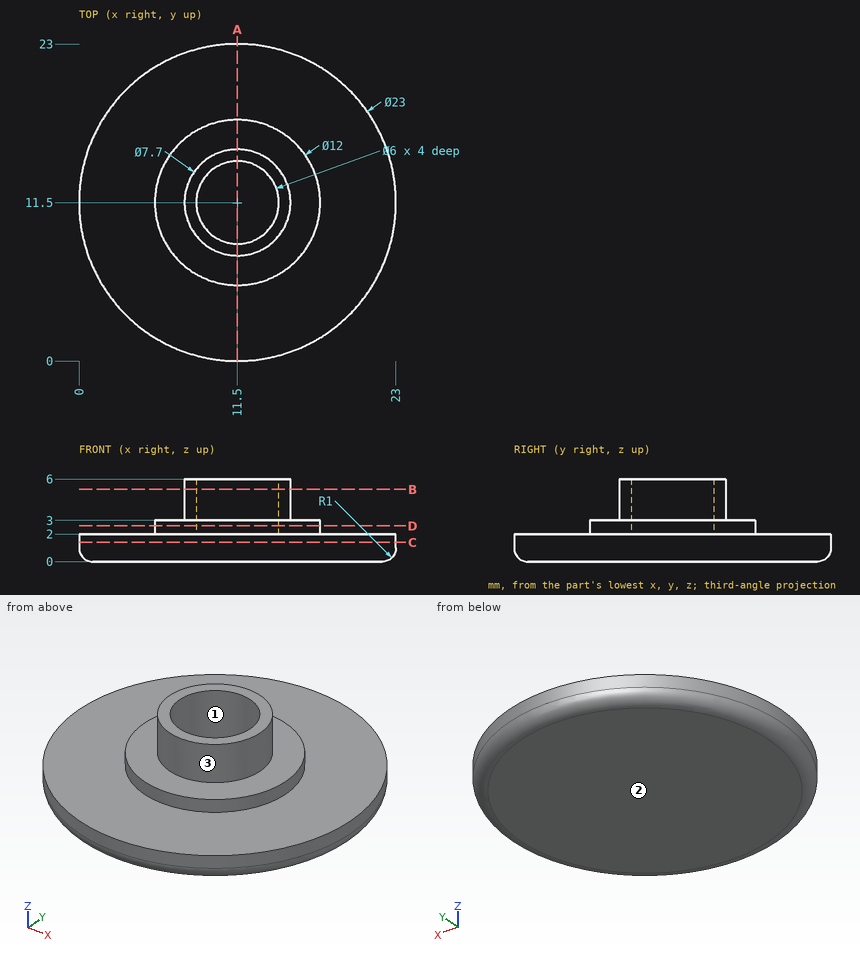
Design review of the part shown in the three views and the two pictorial views. Dimensions are in mm from the part's minimum x, y and z. Give positions to 0.01 mm unless a question says otherwise; leave off trailing zeros. Loops run counter-clockwise (first coordinate to the right, second up) from the corner with the lowest first, then second, coordinate; pieces in that order, holes last. Notation, with made-up numbers: (11, 80.5) -> (29, 80.5) arc R8 ccw to (29, 84.5) -> close; hole circle Ø6 at (72.25, 83). An arc over 180 degrees is marked (long way). One line per item, written item: value.
Q1. We need section B-B on z = 5.25. Give the boundary of the cut face in (x, y).
Numbers:
outline: circle Ø7.7 at (11.5, 11.5); hole circle Ø6 at (11.5, 11.5)
Q2. We need section D-D on z = 2.6. Give the boundary of the cut face in (x, y).
Numbers:
outline: circle Ø12 at (11.5, 11.5); hole circle Ø6 at (11.5, 11.5)
Q3. We need section A-A on x = 11.5. Give the boundary of the cut face in (y, z).
Numbers:
outline: (0, 1) arc R1 ccw to (1, 0) -> (22, 0) arc R1 ccw to (23, 1) -> (23, 2) -> (17.5, 2) -> (17.5, 3) -> (15.35, 3) -> (15.35, 6) -> (14.5, 6) -> (14.5, 2) -> (8.5, 2) -> (8.5, 6) -> (7.65, 6) -> (7.65, 3) -> (5.5, 3) -> (5.5, 2) -> (0, 2) -> close
Q4. For pin 1 Ø3.5 at (x, y) = (10.5, 12) entering from +Z, flat-tipped, find the tip position at first contact; note if it passes through.
Numbers:
pin 1: stops at z = 2
Q5. For L1, parallel to Y at x = 11.5, z = 3.4; L2, parallel to Z at x = 13.5, y = 13.5; L3, parallel to Z at x = 7.5, y = 7.25, list the stretches that pass through material, from the lowest coordinate up.
Numbers:
L1: y = 7.65 to 8.5, 14.5 to 15.35
L2: z = 0 to 2
L3: z = 0 to 3
Q6. Draft analysis for pull direction X (two halves, no side actions). For the marked faces 1, 2 and 3, state which applies: pulls with the +X half, pulls with the -X half, needs draft (parallel to the pull), parting line crosses it, or undercut.
Numbers:
face 1: undercut
face 2: needs draft
face 3: parting line crosses it
Q7. We need section C-C on z = 1.4. Give the boundary of the cut face in (x, y).
Numbers:
outline: circle Ø23 at (11.5, 11.5)
